Check sheet for the drawn part. Datum: minimum x, y, z corner. Units: mm. A direction names the side the tool comes from. Round coordinates to 2 decimals unless told otherwise and drop trailing zeros. Write each loop counter-clockwise with the first axis right and the second up, starting at its lowest first coordinate (ties: lowest second). Pieces come first, ordered by that corner, then holes. Notation, with made-up numbers: M 22.5,-3 L 72.5,-3 A18 cw 72.5,5 Z; hole C -3,77.5 d2. An arc over 180 degrees is marked long. Answer as CSV lines item,"result". Start each with the question number.
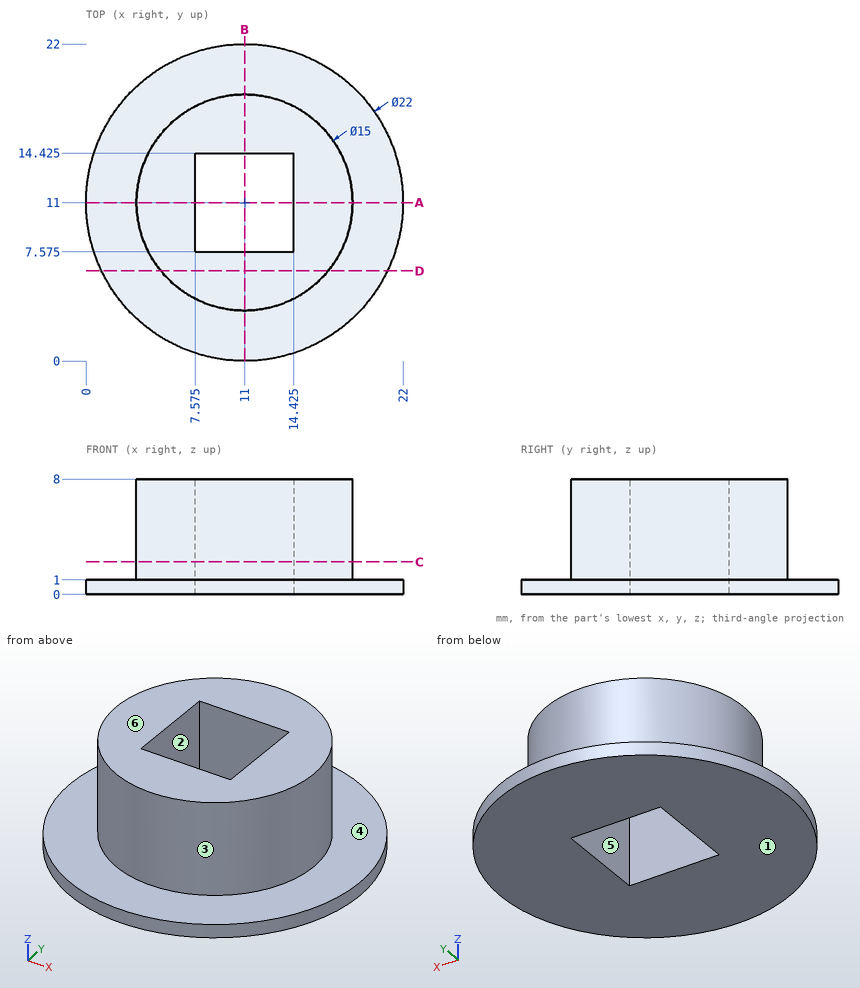
1) Scan lines: line 1 (X direction, y = 11, z = 4.25) (3 decimals); line 2 (Y direction, x = 12.5, z = 3.75) (3 decimals); line 3 (Z direction, x = 8.75, y = 19). Record each from-to range of solid material in increasing order. Write a range as from..to.
2) Go/stop test with flat-tipped pins: pin 1 (1 mm diameter, centred on x = 9, y = 12.5, fed in from -Z); pin 2 (4 mm diameter, centred on y = 17, z = 4.5, fed in from +X); pin 3 (2 mm diameter, centred on x = 11, z = 4, fed in from -Y); pin 4 (1.5 mm diameter, centred on x = 17.5, y = 4, fed in from +Z). Record where each tip stops, or that it passes through.
3) Section check C-C, the plane z = 2.25. Record the cut outline in (x, y) (3 decimals), plus the area to 3 significant figures.
4) Section check D-D, the plane y = 6.25. Record the cut outline in (x, z), plus the area to 3 significant figures.
5) Mould release check, pull along X, two halves, no side actions. Record for the marked faces 1, 2 and 3: released by +X, released by -X, zero draft, split by the parting line, or undercut.
6) Access from +Z, -Z, +X, -X, +Y, -Y to the whole of each face (thin tool, end or side, straight path). Record for the marked faces 4, 5 and 6.
7) Section check A-A, the plane y = 11. Record the cut outline in (x, z) (3 decimals).
Results:
1,line 1,"x = 3.5..7.575, 14.425..18.5"
1,line 2,"y = 3.652..7.575, 14.425..18.348"
1,line 3,"z = 0..1"
2,pin 1,"passes through"
2,pin 2,"stops at x = 17.34"
2,pin 3,"stops at y = 3.5"
2,pin 4,"stops at z = 1"
3,outline,"C 11,11 d15; hole M 7.575,7.575 L 14.425,7.575 L 14.425,14.425 L 7.575,14.425 Z"
3,area,"130 mm^2"
4,outline,"M 1.08,0 L 20.92,0 L 20.92,1 L 16.8,1 L 16.8,8 L 5.2,8 L 5.2,1 L 1.08,1 Z"
4,area,"101 mm^2"
5,face 1,"zero draft"
5,face 2,"undercut"
5,face 3,"split by the parting line"
6,face 4,"+Z"
6,face 5,"+Z, -Z"
6,face 6,"+Z, +X, -X, +Y, -Y"
7,outline,"M 0,0 L 7.575,0 L 7.575,8 L 3.5,8 L 3.5,1 L 0,1 Z; M 14.425,0 L 22,0 L 22,1 L 18.5,1 L 18.5,8 L 14.425,8 Z"
